```python
from build123d import *

# Parameters (mm, degrees)
PAD_DEPTH = 20


with BuildPart() as part:
    # Sketch039 → Revolution002 (revolve)
    with BuildSketch(Plane.YZ):
        Polygon((6.95, 11.5), (6.95, 0), (-4.95, 0), (-4.95, 11.5), (-3.75, 11.5), (-1.75, 9.5), (1.75, 9.5), (3.75, 11.5), (4.95, 11.5), align=None)
    revolve(axis=Axis((0, 0, 0), (0, 1, 0)))

    # Sketch041 (on DatumPlane) → Pad (new body)
    with BuildSketch(Plane(origin=(-3, 4.95, 0), x_dir=(0, 0, 1), z_dir=(0, 1, 0))):
        Polygon((0, 6), (-5.196152, 3), (-5.196152, -3), (0, -6), (5.196152, -3), (5.196152, 3), align=None)
    extrude(amount=PAD_DEPTH)

    # Sketch042 (on DatumPlane) → Groove (revolve, cut)
    with BuildSketch(Plane(origin=(-3, 4.95, 0), x_dir=(0, -1, 0), z_dir=(0, 0, 1))):
        Polygon((-17, 6), (-15, 4), (-13, 6), align=None)
    revolve(axis=Axis((-3, 4.95, 0), (0, -1, 0)), mode=Mode.SUBTRACT)


with BuildPart() as part_1:
    # Body007 placement: moved
    add(part.part.moved(Location((74, -46, 0))))


solid = part_1.part
```
The model under review builds one solid part; all positions refer to its coordinate system, in mm. A direction names the side the tool comes from. Give positions to 0.01 mm unless a question says otherwise; leave off trailing zeros. Write each loop counter-clockwise with the first axis right and the second up, starting at its lowest first coordinate (ties: lowest second). Pieces come first, ordered by that corner, then holes. Notation, with made-up numbers: (-35, 20.5) -> (20, 20.5) arc R34 cw to (20, 50.5) -> close; hole circle Ø1 at (6.5, -7.5). An arc over 180 degrees is marked (long way). Answer in a Markdown table with one row per item.
1) Add section A-A on y = -33.5. State the section outline as (x, z) points.
Worked answers:
| item | result |
|---|---|
| outline | (65, 0) -> (68, -5.2) -> (74, -5.2) -> (77, 0) -> (74, 5.2) -> (68, 5.2) -> close |
2) For L1, parallel to Y at x = 75.25, z = -9.25; L2, parallel to Z at x = 68.25, y = -28.5; L3, parallel to Y at x = 78.5, z = -10, list the stretches that pass through material, from the lowest coordinate up. Write a range as [from, to].
Worked answers:
| item | result |
|---|---|
| L1 | [-50.95, -39.05] |
| L2 | [-5.2, 5.2] |
| L3 | [-50.95, -49.22], [-42.78, -39.05] |
3) Mouldability with a two-part tool opening along Y and no side actions: class faces 4 (the conical face through (64.6, -44.12, -2.09)), 5 (the flat face through (75.5, -33.2, -2.6)), 6 (the conical face through (66.879, -26.175, 0.181)), 7 (the flat face through (71, -21.05, 0)) as +Y half, -Y half, draft (parallel to the pull), parting line (faces both ways), or undercut.
Worked answers:
| item | result |
|---|---|
| face 4 | undercut |
| face 5 | draft |
| face 6 | undercut |
| face 7 | +Y half |
4) Tool access review of faces 1 (the flat face through (71, -23, -5.196)), 2 (the flat face through (71, -33, 5.196)), 3 (the flat face through (66.5, -23, 2.6)): name each direction out of +Z, -Z, +X, -X, +Y, -Y from which nothing blocks a thin tool from reaching the whole face with its end or side.
Worked answers:
| item | result |
|---|---|
| face 1 | -Z, +X, -X, +Y |
| face 2 | +Z, +X, -X, +Y |
| face 3 | +Z, -X, +Y |
5) Clearance check with flat-ended pins moving along their axes: P1, Ø1.9, axis at x = 70, y = -23.5, coming from the -Z side; P2, Ø1.5, axis at x = 66.5, y = -41.5, coming from the +Z side; P3, Ø6.5, axis at x = 70.5, y = -33.5, coming from the +Z side. State where each tip first meets the part, or that it passes through.
Worked answers:
| item | result |
|---|---|
| P1 | z = -5.2 |
| P2 | z = 9.31 |
| P3 | z = 5.2 |
6) Add section B-B on y = -48.25. State the section outline as (x, z) points.
Worked answers:
| item | result |
|---|---|
| outline | circle Ø20 at (74, 0) |
